The model under review builds one solid part; all positions refer to its coordinate system, in mm. Give positions to 0.01 mm unless a question says otherwise; leave off trailing zeros. Order: outer loops, then holes, each group sorted by start corner. A loop starts at its lowest first (then second) coordinate and runs counter-clockwise, first axis right, second up. Notation, with made-up numbers: (39, 71.25) -> (77, 71.25) arc R12 cw to (77, 77.25) -> close; hole circle Ø1 at (66, 36). An arc over 180 degrees is marked (long way). Use one line per item in the form item = value.
```python
from build123d import *

# Parameters (mm, degrees)
MODEL_R                  = 6.5
MODEL_R_2                = 5.25
MODEL_W                  = 165
MODEL_H                  = 32
RESSALTO_EXTRUS_O1_DEPTH = 1.5


with BuildPart() as part:
    # Model → Ressalto-extrusão1 (new body)
    with BuildSketch(Plane.XY):
        Polygon((270.074227849, 25.427113901), (280.074227849, 25.427113901), (280.074227849, 35.427113901), (288.074227849, 35.427113901), (288.074227849, 173.427113901), (280.074227849, 173.427113901), (280.074227849, 183.427113901), (270.074227849, 183.427113901), (270.074227849, 191.427113901), (22.074227849, 191.427113901), (22.074227849, 183.427113901), (12.074227849, 183.427113901), (12.074227849, 173.427113901), (4.074227849, 173.427113901), (4.074227849, 35.427113901), (12.074227849, 35.427113901), (12.074227849, 25.427113901), (22.074227849, 25.427113901), (22.074227849, 17.427113901), (270.074227849, 17.427113901), align=None)
        with Locations((36.574227849, 160.927113901)):
            Circle(MODEL_R, mode=Mode.SUBTRACT)
        with Locations((36.574227849, 136.177113901)):
            Circle(MODEL_R, mode=Mode.SUBTRACT)
        with Locations((93.574227849, 110.927113901)):
            Circle(MODEL_R, mode=Mode.SUBTRACT)
        with Locations((144.574227849, 110.927113901)):
            Circle(MODEL_R, mode=Mode.SUBTRACT)
        with Locations((195.574227849, 110.927113901)):
            Circle(MODEL_R, mode=Mode.SUBTRACT)
        with Locations((195.574227849, 160.927113901)):
            Circle(MODEL_R, mode=Mode.SUBTRACT)
        with Locations((144.574227849, 160.927113901)):
            Circle(MODEL_R, mode=Mode.SUBTRACT)
        with Locations((93.574227849, 160.927113901)):
            Circle(MODEL_R, mode=Mode.SUBTRACT)
        with Locations((246.574227849, 142.427113901)):
            Circle(MODEL_R_2, mode=Mode.SUBTRACT)
        with Locations((259.574227849, 142.427113901)):
            Circle(MODEL_R_2, mode=Mode.SUBTRACT)
        with Locations((259.574227849, 129.427113901)):
            Circle(MODEL_R_2, mode=Mode.SUBTRACT)
        with Locations((246.574227849, 129.427113901)):
            Circle(MODEL_R_2, mode=Mode.SUBTRACT)
        with Locations((142.574227849, 136.177113901)):
            Rectangle(MODEL_W, MODEL_H, mode=Mode.SUBTRACT)
    extrude(amount=RESSALTO_EXTRUS_O1_DEPTH)


solid = part.part
```
1. Add section C-C on z = 1. Count the separate pieces of the cut face and the enclosed holes in it, then the cut area to 3 significant figures.
Values:
separate_pieces = 1
enclosed_holes = 13
area = 41,800 mm^2
2. The part is to be moulded in two halves that separate along X. For faces 1 (the face through (144, 86, 1.5)), 2 (the face through (254.33, 129.66, 0.74)), say which applies: +X half, -X half, draft (parallel to the pull), parting line (faces both ways), or undercut.
Values:
face_1 = draft
face_2 = undercut
3. For pin 1 Ø6 at (x, y) = (60, 59) entering from -Z; pin 2 Ø0.8 at (x, z) = (285, 1) entering from +Y, all flat-tipped, find the tip position at first contact; note any pin that passes through.
Values:
pin_1 = 0
pin_2 = 173.43
4. Add section B-B on x = 93.5. Give the boundary of the cut face in (y, z), then the cut area to 3 significant figures.
Values:
outline = (17.43, 0) -> (104.43, 0) -> (104.43, 1.5) -> (17.43, 1.5) -> close; (117.43, 0) -> (120.18, 0) -> (120.18, 1.5) -> (117.43, 1.5) -> close; (152.18, 0) -> (154.43, 0) -> (154.43, 1.5) -> (152.18, 1.5) -> close; (167.43, 0) -> (191.43, 0) -> (191.43, 1.5) -> (167.43, 1.5) -> close
area = 174 mm^2
5. For L1, parallel to X at y = 111, z = 1.3; L2, parallel to Y at x = 247, z = 0.8; L3, parallel to Y at x = 151.5, z = 0.9, list the stretches that pass through material, from the lowest coordinate up.
Values:
L1 = 4.07 to 87.07, 100.07 to 138.07, 151.07 to 189.07, 202.07 to 288.07
L2 = 17.43 to 124.19, 134.66 to 137.19, 147.66 to 191.43
L3 = 17.43 to 120.18, 152.18 to 191.43
6. Add section A-A on x = 205. Give the boundary of the cut face in (y, z).
Values:
outline = (17.43, 0) -> (120.18, 0) -> (120.18, 1.5) -> (17.43, 1.5) -> close; (152.18, 0) -> (191.43, 0) -> (191.43, 1.5) -> (152.18, 1.5) -> close
